Part model, mm, in its own coordinate system. Give positions to 0.01 mm unless a question says otherwise; leave off trailing zeros. Order: outer loops, then holes, each group sorted by start corner. A loop starts at its lowest first (then second) coordinate and runs counter-clockwise, first axis right, second up. Notation, with made-up numbers: (77.25, 65.5) - (84.25, 65.5) arc R17 ccw to (84.25, 71.5) - close; hole circle Ø11 at (55.5, 58.25). An arc over 180 degrees is marked (long way). One line per item, written item: value.
```python
from build123d import *

# Parameters (mm, degrees)
SKETCH1_R           = 27.94
BOSS_EXTRUDE1_DEPTH = 20.32
SKETCH2_R           = 6.35
BOSS_EXTRUDE2_DEPTH = 20.32
BOSS_EXTRUDE3_START = 20.32
SKETCH3_R           = 27.94
BOSS_EXTRUDE3_DEPTH = 20.32
FILLET1_R           = 5.08
FILLET2_R           = 5.08
FILLET3_R           = 5.08
FILLET4_R           = 5.08
CUT_EXTRUDE1_DEPTH  = 73.645776241
SKETCH6_R           = 27.94
CUT_EXTRUDE2_DEPTH  = 57.682420605
SKETCH7_R           = 6.35
CUT_EXTRUDE3_DEPTH  = 5.08
SKETCH9_R           = 6.35
CUT_EXTRUDE5_DEPTH  = 10.16
SKETCH10_W          = 5.08
SKETCH10_H          = 5.08
BOSS_EXTRUDE4_DEPTH = 12.7


with BuildPart() as part:
    # Sketch1 → Boss-Extrude1 (new body)
    with BuildSketch(Plane.XY):
        Circle(SKETCH1_R)
    extrude(amount=BOSS_EXTRUDE1_DEPTH)

    # Sketch2 → Boss-Extrude2 (add)
    with BuildSketch(Plane(origin=(0, 0, 0), x_dir=(-1, 0, 0), z_dir=(0, 0, -1))):
        with Locations(Location((0, 0, 0), (0, 0, 180))):
            Circle(SKETCH2_R)
    extrude(amount=BOSS_EXTRUDE2_DEPTH)

    # Sketch3 → Boss-Extrude3 (add)
    with BuildSketch(Plane(origin=(0, 0, -20.32), x_dir=(-1, 0, 0), z_dir=(0, 0, -1)).offset(BOSS_EXTRUDE3_START)):
        with Locations(Location((0, 0, 0), (0, 0, 180))):
            Circle(SKETCH3_R)
    extrude(amount=-BOSS_EXTRUDE3_DEPTH)

    # Fillet1
    fillet1_edges = [part.edges().sort_by_distance(p)[0] for p in [
        (-27.94, 0, 20.32),
    ]]
    fillet(fillet1_edges, radius=FILLET1_R)

    # Fillet2
    fillet2_edges = [part.edges().sort_by_distance(p)[0] for p in [
        (-27.94, 0, 0),
    ]]
    fillet(fillet2_edges, radius=FILLET2_R)

    # Fillet3
    fillet3_edges = [part.edges().sort_by_distance(p)[0] for p in [
        (-27.94, 0, -20.32),
    ]]
    fillet(fillet3_edges, radius=FILLET3_R)

    # Fillet4
    fillet4_edges = [part.edges().sort_by_distance(p)[0] for p in [
        (-27.94, 0, -40.64),
    ]]
    fillet(fillet4_edges, radius=FILLET4_R)

    # Sketch4 → Cut-Extrude1 (cut, through all)
    with BuildSketch(Plane(origin=(0, 0, -40.64), x_dir=(-1, 0, 0), z_dir=(0, 0, -1))):
        with BuildLine():
            Line((-3.556, 8.739962471), (-3.556, 17.568282329))
            ThreePointArc((-3.556, 17.568282329), (-5.256117539, 20.740741312), (-8.8392, 21.081938795))
            ThreePointArc((-8.8392, 21.081938795), (-19.797340731, 11.43), (-22.677094558, -2.885997648))
            ThreePointArc((-22.677094558, -2.885997648), (-20.590067639, -5.818439342), (-16.992578798, -5.704554829))
            Line((-16.992578798, -5.704554829), (-9.347029528, -1.2903949))
            ThreePointArc((-9.347029528, -1.2903949), (-8.133427478, -0.179541209), (-7.501353019, 1.339441259))
            ThreePointArc((-7.501353019, 1.339441259), (-6.599113577, 3.81), (-4.910666667, 5.826641648))
            ThreePointArc((-4.910666667, 5.826641648), (-3.911226491, 7.13352542), (-3.556, 8.739962471))
        make_face()
        with BuildLine():
            Line((3.556, 8.739962471), (3.556, 17.568282329))
            ThreePointArc((3.556, 17.568282329), (5.256117539, 20.740741312), (8.8392, 21.081938795))
            ThreePointArc((8.8392, 21.081938795), (19.797340731, 11.43), (22.677094558, -2.885997648))
            ThreePointArc((22.677094558, -2.885997648), (20.590067639, -5.818439342), (16.992578798, -5.704554829))
            Line((16.992578798, -5.704554829), (9.347029528, -1.2903949))
            ThreePointArc((9.347029528, -1.2903949), (8.133427478, -0.179541209), (7.501353019, 1.339441259))
            ThreePointArc((7.501353019, 1.339441259), (6.599113577, 3.81), (4.910666667, 5.826641648))
            ThreePointArc((4.910666667, 5.826641648), (3.911226491, 7.13352542), (3.556, 8.739962471))
        make_face()
        with BuildLine():
            Line((5.791029528, -7.449567572), (13.436578798, -11.8637275))
            ThreePointArc((13.436578798, -11.8637275), (15.3339501, -14.92230197), (13.837894558, -18.195941147))
            ThreePointArc((13.837894558, -18.195941147), (0, -22.86), (-13.837894558, -18.195941147))
            ThreePointArc((-13.837894558, -18.195941147), (-15.3339501, -14.92230197), (-13.436578798, -11.8637275))
            Line((-13.436578798, -11.8637275), (-5.791029528, -7.449567572))
            ThreePointArc((-5.791029528, -7.449567572), (-4.222200987, -6.953984211), (-2.590686352, -7.166082907))
            ThreePointArc((-2.590686352, -7.166082907), (0, -7.62), (2.590686352, -7.166082907))
            ThreePointArc((2.590686352, -7.166082907), (4.222200987, -6.953984211), (5.791029528, -7.449567572))
        make_face()
    extrude(amount=-CUT_EXTRUDE1_DEPTH, mode=Mode.SUBTRACT)

    # Sketch6 → Cut-Extrude2 (cut, through all)
    with BuildSketch(Plane(origin=(0, 0, 0), x_dir=(-1, 0, 0), z_dir=(0, 0, -1))):
        Circle(SKETCH6_R)
    extrude(amount=-CUT_EXTRUDE2_DEPTH, mode=Mode.SUBTRACT)

    # Sketch7 → Cut-Extrude3 (cut)
    with BuildSketch(Plane.XY):
        Circle(SKETCH7_R)
    extrude(amount=-CUT_EXTRUDE3_DEPTH, mode=Mode.SUBTRACT)

    # Sketch9 → Cut-Extrude5 (cut)
    with BuildSketch(Plane.XY.offset(-5.08)):
        Circle(SKETCH9_R)
    extrude(amount=-CUT_EXTRUDE5_DEPTH, mode=Mode.SUBTRACT)

    # Sketch10 → Boss-Extrude4 (add)
    with BuildSketch(Plane.XY.offset(-15.24)):
        Rectangle(SKETCH10_W, SKETCH10_H)
    extrude(amount=BOSS_EXTRUDE4_DEPTH)


solid = part.part
```
1) Cut at D-D, the plane z = -11. Give the cut face in (x, y), then the cut area to 3 significant figures.
Outcome:
outline: (-2.54, -2.54) - (2.54, -2.54) - (2.54, 2.54) - (-2.54, 2.54) - close
area: 25.8 mm^2
2) Cut at C-C, the plane y = 0. Give the cut face in (x, z), then the cut area to 3 significant figures.
Outcome:
outline: (-27.94, -35.56) arc R5.08 ccw to (-22.86, -40.64) - (-22.86, -20.32) arc R5.08 ccw to (-27.94, -25.4) - close; (-8.01, -40.64) - (8.01, -40.64) - (8.01, -20.32) - (6.35, -20.32) - (6.35, -15.24) - (2.54, -15.24) - (2.54, -2.54) - (-2.54, -2.54) - (-2.54, -15.24) - (-6.35, -15.24) - (-6.35, -20.32) - (-8.01, -20.32) - close; (22.86, -40.64) arc R5.08 ccw to (27.94, -35.56) - (27.94, -25.4) arc R5.08 ccw to (22.86, -20.32) - close
area: 639 mm^2
3) Mould opens along X. For faces 1 (the cylindrical face through (-4.199, -6.952, -30.622)), 2 (the flat face through (0, 0, -2.54)), 3 (the cylindrical face through (2.93, 5.634, -17.744)), 4 (the cylindrical face through (8.15, -0.2, -30.62)) say: released by +X, released by -X, zero draft, split by the parting line, or undercut.
Outcome:
face 1: undercut
face 2: zero draft
face 3: split by the parting line
face 4: undercut
4) Drill centre lines: line 1 along X through (y, z) = (0.5, -26.5); line 2 along Y through (x, z) = (-4.5, -33); line 3 along X through (y, z) = (17, -28.5). Where is each one in solid material? Low to high. Write a range as from..to.
Outcome:
line 1: x = -27.94..-22.85, -7.75..7.75, 22.85..27.94
line 2: y = -27.58..-22.41, -6.99..6.23, 20.08..27.58
line 3: x = -22.17..-15.28, -3.56..3.56, 15.28..22.17
5) Pin check, flat tips, straight feed: pin 1 (1 mm diameter, centred on y = -18, z = -26, fed in from -X); pin 2 (4 mm diameter, centred on y = -0.5, z = -9.5, fed in from -X); pin 3 (1 mm diameter, centred on y = -5.5, z = -34, fed in from +X). Stop position of each tip, or through.
Outcome:
pin 1: stops at x = -21.78
pin 2: stops at x = -2.54
pin 3: stops at x = 27.49
6) Cut at B-B, the plane z = -34.5. Give the cut face in (x, y) (3 decimals), then the cut area to 3 significant figures.
Outcome:
outline: circle Ø55.88 at (0, 0); hole (-22.677, -2.886) arc R3.81 ccw to (-16.993, -5.705) - (-9.347, -1.29) arc R3.81 ccw to (-7.501, 1.339) arc R7.62 cw to (-4.911, 5.827) arc R3.81 ccw to (-3.556, 8.74) - (-3.556, 17.568) arc R3.81 ccw to (-8.839, 21.082) arc R22.86 ccw to start; hole (-13.838, -18.196) arc R22.86 ccw to (13.838, -18.196) arc R3.81 ccw to (13.437, -11.864) - (5.791, -7.45) arc R3.81 ccw to (2.591, -7.166) arc R7.62 cw to (-2.591, -7.166) arc R3.81 ccw to (-5.791, -7.45) - (-13.437, -11.864) arc R3.81 ccw to start; hole (3.556, 8.74) arc R3.81 ccw to (4.911, 5.827) arc R7.62 cw to (7.501, 1.339) arc R3.81 ccw to (9.347, -1.29) - (16.993, -5.705) arc R3.81 ccw to (22.677, -2.886) arc R22.86 ccw to (8.839, 21.082) arc R3.81 ccw to (3.556, 17.568) - close
area: 1,360 mm^2
7) Cut at A-A, the plane x = 0. Give the cut face in (y, z), then the cut area to 3 significant figures.
Outcome:
outline: (-27.94, -35.56) arc R5.08 ccw to (-22.86, -40.64) - (-22.86, -20.32) arc R5.08 ccw to (-27.94, -25.4) - close; (-7.62, -40.64) - (22.86, -40.64) arc R5.08 ccw to (27.94, -35.56) - (27.94, -25.4) arc R5.08 ccw to (22.86, -20.32) - (6.35, -20.32) - (6.35, -15.24) - (2.54, -15.24) - (2.54, -2.54) - (-2.54, -2.54) - (-2.54, -15.24) - (-6.35, -15.24) - (-6.35, -20.32) - (-7.62, -20.32) - close
area: 933 mm^2
